```python
from build123d import *

# Parameters (mm, degrees)
BOSS_EXTRUDE2_DEPTH = 10
SKETCH4_R           = 7
CUT_EXTRUDE2_DEPTH  = 10


with BuildPart() as part:
    # Sketch3 → Boss-Extrude2 (new body)
    with BuildSketch(Plane(origin=(0, 0, 0), x_dir=(0, 0, -1), z_dir=(1, 0, 0))):
        with BuildLine():
            Line((-168.70292887, 0), (191.29707113, 0))
            ThreePointArc((191.29707113, 0), (11.29707113, 180), (-168.70292887, 0))
        make_face()
    extrude(amount=BOSS_EXTRUDE2_DEPTH)

    # Sketch4 → Cut-Extrude2 (cut)
    with BuildSketch(Plane.ZY):
        with Locations((-160.781790175, 25)):
            Circle(SKETCH4_R)
        with Locations((-135.781790175, 25)):
            Circle(SKETCH4_R)
        with Locations((-110.781790175, 25)):
            Circle(SKETCH4_R)
        with Locations((-85.781790175, 25)):
            Circle(SKETCH4_R)
        with Locations((-60.781790175, 25)):
            Circle(SKETCH4_R)
        with Locations((-35.781790175, 25)):
            Circle(SKETCH4_R)
        with Locations((-10.781790175, 25)):
            Circle(SKETCH4_R)
        with Locations((14.218209825, 25)):
            Circle(SKETCH4_R)
        with Locations((39.218209825, 25)):
            Circle(SKETCH4_R)
        with Locations((64.218209825, 25)):
            Circle(SKETCH4_R)
        with Locations((89.218209825, 25)):
            Circle(SKETCH4_R)
        with Locations((114.218209825, 25)):
            Circle(SKETCH4_R)
        with Locations((139.218209825, 25)):
            Circle(SKETCH4_R)
        with Locations((-135.781790175, 50)):
            Circle(SKETCH4_R)
        with Locations((-110.781790175, 50)):
            Circle(SKETCH4_R)
        with Locations((-85.781790175, 50)):
            Circle(SKETCH4_R)
        with Locations((-60.781790175, 50)):
            Circle(SKETCH4_R)
        with Locations((-35.781790175, 50)):
            Circle(SKETCH4_R)
        with Locations((-10.781790175, 50)):
            Circle(SKETCH4_R)
        with Locations((14.218209825, 50)):
            Circle(SKETCH4_R)
        with Locations((39.218209825, 50)):
            Circle(SKETCH4_R)
        with Locations((64.218209825, 50)):
            Circle(SKETCH4_R)
        with Locations((89.218209825, 50)):
            Circle(SKETCH4_R)
        with Locations((114.218209825, 50)):
            Circle(SKETCH4_R)
        with Locations((139.218209825, 50)):
            Circle(SKETCH4_R)
        with Locations((-135.781790175, 75)):
            Circle(SKETCH4_R)
        with Locations((-110.781790175, 75)):
            Circle(SKETCH4_R)
        with Locations((-85.781790175, 75)):
            Circle(SKETCH4_R)
        with Locations((-60.781790175, 75)):
            Circle(SKETCH4_R)
        with Locations((-35.781790175, 75)):
            Circle(SKETCH4_R)
        with Locations((-10.781790175, 75)):
            Circle(SKETCH4_R)
        with Locations((14.218209825, 75)):
            Circle(SKETCH4_R)
        with Locations((39.218209825, 75)):
            Circle(SKETCH4_R)
        with Locations((64.218209825, 75)):
            Circle(SKETCH4_R)
        with Locations((89.218209825, 75)):
            Circle(SKETCH4_R)
        with Locations((114.218209825, 75)):
            Circle(SKETCH4_R)
        with Locations((139.218209825, 75)):
            Circle(SKETCH4_R)
        with Locations((-135.781790175, 100)):
            Circle(SKETCH4_R)
        with Locations((-110.781790175, 100)):
            Circle(SKETCH4_R)
        with Locations((-85.781790175, 100)):
            Circle(SKETCH4_R)
        with Locations((-60.781790175, 100)):
            Circle(SKETCH4_R)
        with Locations((-35.781790175, 100)):
            Circle(SKETCH4_R)
        with Locations((-10.781790175, 100)):
            Circle(SKETCH4_R)
        with Locations((14.218209825, 100)):
            Circle(SKETCH4_R)
        with Locations((39.218209825, 100)):
            Circle(SKETCH4_R)
        with Locations((64.218209825, 100)):
            Circle(SKETCH4_R)
        with Locations((89.218209825, 100)):
            Circle(SKETCH4_R)
        with Locations((114.218209825, 100)):
            Circle(SKETCH4_R)
        with Locations((-110.781790175, 125)):
            Circle(SKETCH4_R)
        with Locations((-85.781790175, 125)):
            Circle(SKETCH4_R)
        with Locations((-60.781790175, 125)):
            Circle(SKETCH4_R)
        with Locations((-35.781790175, 125)):
            Circle(SKETCH4_R)
        with Locations((-10.781790175, 125)):
            Circle(SKETCH4_R)
        with Locations((14.218209825, 125)):
            Circle(SKETCH4_R)
        with Locations((39.218209825, 125)):
            Circle(SKETCH4_R)
        with Locations((64.218209825, 125)):
            Circle(SKETCH4_R)
        with Locations((89.218209825, 125)):
            Circle(SKETCH4_R)
        with Locations((-85.781790175, 150)):
            Circle(SKETCH4_R)
        with Locations((-60.781790175, 150)):
            Circle(SKETCH4_R)
        with Locations((-35.781790175, 150)):
            Circle(SKETCH4_R)
        with Locations((-10.781790175, 150)):
            Circle(SKETCH4_R)
        with Locations((14.218209825, 150)):
            Circle(SKETCH4_R)
        with Locations((39.218209825, 150)):
            Circle(SKETCH4_R)
        with Locations((64.218209825, 150)):
            Circle(SKETCH4_R)
        with Locations((-160.781790175, 50)):
            Circle(SKETCH4_R)
        with Locations((-160.781790175, 75)):
            Circle(SKETCH4_R)
    extrude(amount=-CUT_EXTRUDE2_DEPTH, mode=Mode.SUBTRACT)


solid = part.part
```
Geometry check sheet. Reference: the model listing, model coordinates, mm. Round coordinates to 2 decimals unless told otherwise and drop trailing zeros. Order: outer loops, then holes, each group sorted by start corner. A loop starts at its lowest first (then second) coordinate and runs counter-clockwise, first axis right, second up. Notation, with made-up numbers: M 86,77 L 124,77 A22 ccw 124,100 Z; hole C 47,-32.75 d1. An arc over 180 degrees is marked long. Write item = value, one per line.
Q1. Depth check by flat-ended pin: pin 1 Ø1.5 at (x, y) = (3.5, 94.5) entering from +Z; pin 2 Ø8.5 at (y, z) = (25, -160.78) entering from +X; pin 3 Ø3 at (x, z) = (4.5, -123.5) entering from +Y; pin 4 Ø5 at (x, y) = (1, 83.5) entering from -Z. Enter the tip coordinate at first touch or a pass-through.
Answer block:
pin_1 = 142.36
pin_2 = through
pin_3 = 141.93
pin_4 = -172.04
Q2. Section check B-B (y = 150). Give the number of separate pieces and of enclosed holes in the cut face, plus the area to 3 significant figures.
Answer block:
separate_pieces = 8
enclosed_holes = 0
area = 1,010 mm^2
Q3. Section check A-A (z = -87). Enter the section's corners in (x, y), plus the area to 3 significant figures.
Answer block:
outline = M 0,0 L 10,0 L 10,18.11 L 0,18.11 Z; M 0,31.89 L 10,31.89 L 10,43.11 L 0,43.11 Z; M 0,56.89 L 10,56.89 L 10,68.11 L 0,68.11 Z; M 0,81.89 L 10,81.89 L 10,93.11 L 0,93.11 Z; M 0,106.89 L 10,106.89 L 10,118.11 L 0,118.11 Z; M 0,131.89 L 10,131.89 L 10,143.11 L 0,143.11 Z; M 0,156.89 L 10,156.89 L 10,163.31 L 0,163.31 Z
area = 806 mm^2
Q4. Scan lines: line 1 (Y direction, x = 4.25, z = 140.5); line 2 (Y direction, x = 1, z = -141.5); line 3 (Y direction, x = 3.5, z = 140). Record each from-to range of solid material in increasing order.
Answer block:
line_1 = 0 to 18.12, 31.88 to 43.12, 56.88 to 68.12, 81.88 to 96.73
line_2 = 0 to 20.96, 29.04 to 45.96, 54.04 to 70.96, 79.04 to 95.96, 104.04 to 124.29
line_3 = 0 to 18.04, 31.96 to 43.04, 56.96 to 68.04, 81.96 to 97.52
Q5. Release check for a two-part mould opening along Y. For faces 1 (the cylindrical face through (4.93, 143.79, 67.45)), 2 (the flat face through (10, 91, -9)) record: released by +Y, released by -Y, zero draft, split by the parting line, or undercut.
Answer block:
face_1 = undercut
face_2 = zero draft
